```python
from build123d import *

# Parameters (mm, degrees)
SKETCH1_R           = 5
BOSS_EXTRUDE1_DEPTH = 8
SKETCH2_R           = 8
CUT_EXTRUDE1_DEPTH  = 5
SKETCH3_W           = 25
SKETCH3_H           = 8
BOSS_EXTRUDE2_DEPTH = 15
SKETCH4_R           = 2.5
CUT_EXTRUDE2_DEPTH  = 10


with BuildPart() as part:
    # Sketch1 → Boss-Extrude1 (new body)
    with BuildSketch(Plane(origin=(0, 0, 0), x_dir=(1, 0, 0), z_dir=(0, 1, 0))):
        with BuildLine():
            Line((-16.25, 12.5), (16.25, 12.5))
            Line((16.25, 12.5), (31.25, 12.5))
            ThreePointArc((31.25, 12.5), (43.75, 0), (31.25, -12.5))
            Line((31.25, -12.5), (16.25, -12.5))
            Line((16.25, -12.5), (-16.25, -12.5))
            Line((-16.25, -12.5), (-16.25, 12.5))
        make_face()
        with Locations((31.25, 0)):
            Circle(SKETCH1_R, mode=Mode.SUBTRACT)
        with BuildLine():
            Line((16.25, 9.5), (16.25, -9.5))
            Line((16.25, -9.5), (23.125961595, -9.5))
            ThreePointArc((23.125961595, -9.5), (18.75, 0), (23.125961595, 9.5))
            Line((23.125961595, 9.5), (16.25, 9.5))
        make_face(mode=Mode.SUBTRACT)
    extrude(amount=BOSS_EXTRUDE1_DEPTH)

    # Sketch2 → Cut-Extrude1 (cut)
    with BuildSketch(Plane(origin=(0, 8, 0), x_dir=(1, 0, 0), z_dir=(0, 1, 0))):
        with Locations((31.25, 0)):
            Circle(SKETCH2_R)
    extrude(amount=-CUT_EXTRUDE1_DEPTH, mode=Mode.SUBTRACT)

    # Sketch3 → Boss-Extrude2 (add)
    with BuildSketch(Plane.ZY.offset(16.25)):
        with Locations((0, 4)):
            Rectangle(SKETCH3_W, SKETCH3_H)
    extrude(amount=BOSS_EXTRUDE2_DEPTH)

    # Sketch4 → Cut-Extrude2 (cut)
    with BuildSketch(Plane(origin=(0, 0, 0), x_dir=(-1, 0, 0), z_dir=(0, -1, 0))):
        with Locations((-0.25, 0)):
            Circle(SKETCH4_R)
        with Locations((19.75, 0)):
            Circle(SKETCH4_R)
    extrude(amount=-CUT_EXTRUDE2_DEPTH, mode=Mode.SUBTRACT)


solid = part.part
```
Geometry: final body of the model. Coordinates: model frame, mm. A direction names the side the tool comes from. Coordinates: 2 decimals unless noted, no trailing zeros. Order: outer loops, then holes, each group sorted by start corner. A loop starts at its lowest first (then second) coordinate and runs counter-clockwise, first axis right, second up. Notation, with made-up numbers: M 28.5,-4 L 50.5,-4 A31 ccw 50.5,21 Z; hole C -27,70.5 d10. An arc over 180 degrees is marked long. Answer in a Markdown table with one row per item. Add a question column.
Q1. Reachability of faces 4 (the flat face through (16.25, 4, 0)), 5 (the cylindrical face through (23.258, 5.535, -0.352)), 6 (the flat face through (7, 8, 0)) from +Z, -Z, +X, -X, +Y, -Y: full face, straight path, thin tool, end or side. Return the list, or none.
Q2. Section query C-C on z = 0. Return the cut outline in (x, y).
Q3. Line query: L1, parallel to Z at x = -19.75, y = 4.25; L2, parallel to X at y = 1.75, z = 2.25; L3, parallel to Z at x = 31.25, y = 1. Output: solid intervals per line, ascending.
Q4. Section query B-B on y = 1.5. Return the cut outline in (x, z), and give its area (3 significant figures).
Q5. Contact query for flat-ended pins moving along their axis: P1, Ø1.5, axis at y = 2.5, z = 4.5, coming from the +X side; P2, Ø8, axis at x = 32, z = -1.5, coming from the +Y side; P3, Ø4, axis at y = 4, z = -2.5, coming from the +X side. Output: stop coordinate, or through.
Q6. Section query D-D on z = 3.25. Return the cut outline in (x, y).
Q7. Mould query, pull axis Z, two halves, no side actions, for faces 1 (the flat face through (20, 4, 9.5)), 2 (the flat face through (0, 4, -12.5)), 3 (the flat face through (0, 4, 12.5)). Classes: released by +Z, released by -Z, zero draft, split by the parting line, or undercut.
Q8. Section query A-A on x = -19.75. Return the cut outline in (y, z).
Completed:
| question | item | result |
|---|---|---|
| 1 | face 4 | +Y, -Y |
| 1 | face 5 | +Y |
| 1 | face 6 | +Z, -Z, +X, -X, +Y |
| 2 | outline | M -31.25,0 L -22.25,0 L -22.25,8 L -31.25,8 Z; M -17.25,0 L -2.25,0 L -2.25,8 L -17.25,8 Z; M 2.75,0 L 16.25,0 L 16.25,8 L 2.75,8 Z; M 18.75,0 L 26.25,0 L 26.25,3 L 23.25,3 L 23.25,8 L 18.75,8 Z; M 36.25,0 L 43.75,0 L 43.75,8 L 39.25,8 L 39.25,3 L 36.25,3 Z |
| 3 | L1 | z = -12.5 to -2.5, 2.5 to 12.5 |
| 3 | L2 | x = -31.25 to -20.84, -18.66 to -0.84, 1.34 to 16.25, 18.95 to 26.78, 35.72 to 43.55 |
| 3 | L3 | z = -12.5 to -5, 5 to 12.5 |
| 4 | outline | M -31.25,-12.5 L 31.25,-12.5 A12.5 ccw 31.25,12.5 L -31.25,12.5 Z; hole C -19.75,0 d5; hole C 0.25,0 d5; hole M 16.25,-9.5 L 23.13,-9.5 A12.5 cw 23.13,9.5 L 16.25,9.5 Z; hole C 31.25,0 d10 |
| 4 | area | 1,620 mm2 |
| 5 | P1 | stops at x = 43.17 |
| 5 | P2 | stops at y = 3 |
| 5 | P3 | stops at x = 43.74 |
| 6 | outline | M -31.25,0 L 16.25,0 L 16.25,8 L -31.25,8 Z; M 19.18,0 L 27.45,0 L 27.45,3 L 23.94,3 L 23.94,8 L 19.18,8 Z; M 35.05,0 L 43.32,0 L 43.32,8 L 38.56,8 L 38.56,3 L 35.05,3 Z |
| 7 | face 1 | undercut |
| 7 | face 2 | released by -Z |
| 7 | face 3 | released by +Z |
| 8 | outline | M 0,-12.5 L 8,-12.5 L 8,-2.5 L 0,-2.5 Z; M 0,2.5 L 8,2.5 L 8,12.5 L 0,12.5 Z |
